Part print with two shaded views. Sizes in mm from the minimum x, y, z corner. Give positions to 0.01 mm unless a question says otherwise; leave off trailing zeros. Write each loop counter-clockwise with the first axis right and the second up, starting at its lowest first coordinate (ties: lowest second). Pieces come first, ordered by that corner, then holes. Notation, with made-up numbers: (9.25, -12) -> (68.25, -12) arc R11 ccw to (68.25, -8) -> close; hole circle Ø6 at (17, 3.25). An arc over 180 degrees is marked (long way). Answer as a JSON object with one key per item and string values.
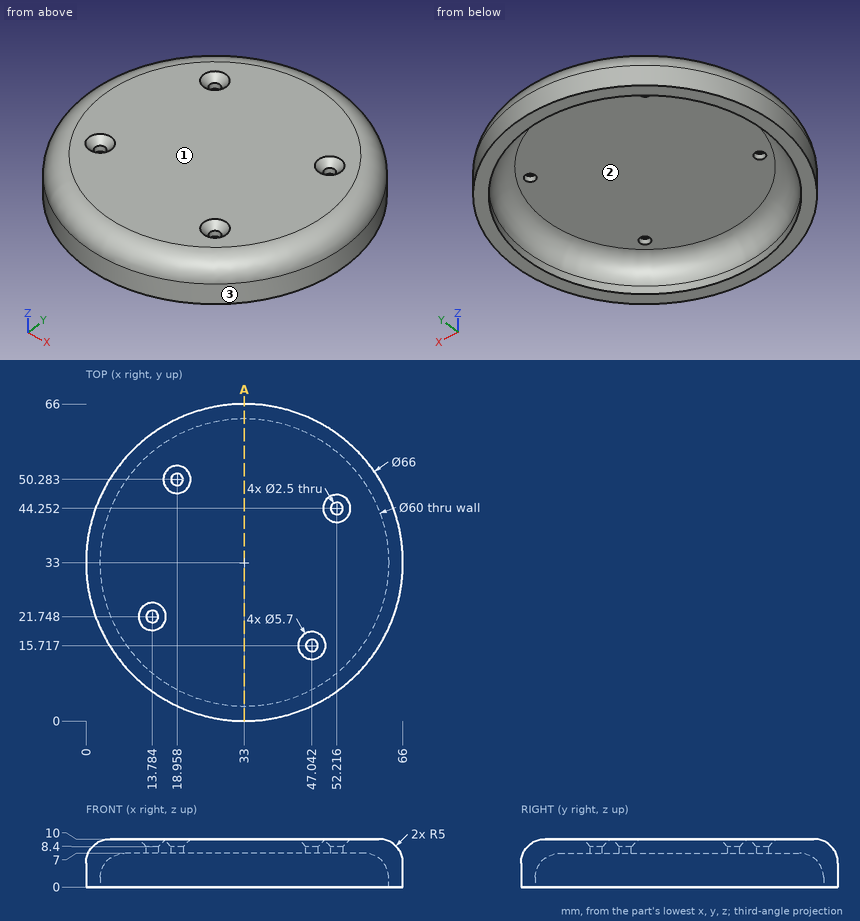
1) Pin check, flat tips, straight feed: pin 1 (3 mm diameter, centred on x = 9, z = 6.5, fed in from +Y); pin 2 (4 mm diameter, centred on y = 14, z = 7, fed in from +X); pin 3 (1.5 mm diameter, centred on y = 58, z = 6, fed in from -X). Stop position of each tip, or through.
Model answer:
{"pin 1": "stops at y = 56.92", "pin 2": "stops at x = 61.01", "pin 3": "stops at x = 10.74"}
2) Mould opens along X. For the marked faces 1, 2 and 3 say: released by +X, released by -X, zero draft, split by the parting line, or undercut.
Model answer:
{"face 1": "zero draft", "face 2": "undercut", "face 3": "split by the parting line"}
3) Slice it at A-A (x = 33). List the corners of the cut face in (y, z), then the cut area to 3 significant figures.
Model answer:
{"outline": "(0, 0) -> (3, 0) -> (3, 2) arc R5 cw to (8, 7) -> (58, 7) arc R5 cw to (63, 2) -> (63, 0) -> (66, 0) -> (66, 5) arc R5 ccw to (61, 10) -> (5, 10) arc R5 ccw to (0, 5) -> close", "area": "240 mm2"}
4) Wall check: probe 1 along Z at (x, y) = (17.5, 31); probe 2 along Y at (x, z) = (27.5, 2.75) (1 decimal); probe 3 along X at (y, z) = (10.5, 3.25) (1 decimal). Give the ranges that are in metal, low to high.
Model answer:
{"probe 1": "z = 7 to 10", "probe 2": "y = 0.5 to 3.6, 62.4 to 65.5", "probe 3": "x = 8.9 to 13.4, 52.6 to 57.1"}
